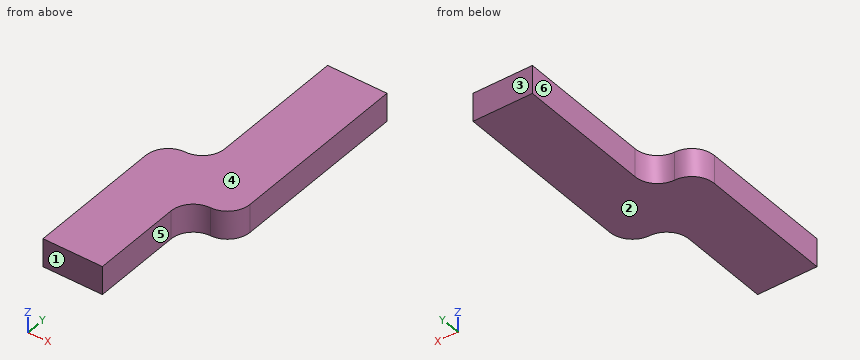
from build123d import *

# Parameters (mm, degrees)
F1_DEPTH = 6.3


with BuildPart() as f1:
    # F0 (on Top) → F1 (new body)
    with BuildSketch(Plane.XY):
        with BuildLine():
            Line((0, 30), (0, 0))
            Line((0, 0), (13.2, 0))
            Line((13.2, 0), (13.2, 20))
            ThreePointArc((13.2, 20), (14.664466, 23.535534), (18.2, 25))
            ThreePointArc((18.2, 25), (21.735534, 26.464466), (23.2, 30))
            Line((23.2, 30), (23.2, 70))
            Line((23.2, 70), (10, 70))
            Line((10, 70), (10, 40))
            ThreePointArc((10, 40), (8.535534, 36.464466), (5, 35))
            ThreePointArc((5, 35), (1.464466, 33.535534), (0, 30))
        make_face()
    extrude(amount=F1_DEPTH)


solid = f1.part
The listing builds one solid part. Answer for the finished solid, in the listing's coordinates (mm). Face numbers are marked on the shaded views. A direction names the side the tool comes from. Give positions to 0.01 mm unless a question says otherwise; leave off trailing zeros. Loops run counter-clockwise (first coordinate to the right, second up) from the corner with the lowest first, then second, coordinate; pieces in that order, holes last. Notation, with made-up numbers: (23, 5.25) - (61, 5.25) arc R11 ccw to (61, 10.25) - close; hole circle Ø5 at (0, 3.5). An arc over 180 degrees is marked (long way). Use one line per item in the form item = value.
1. Which of the six approach directions +Z, -Z, +X, -X, +Y, -Y give full straight-line access (tool end or side, diameter ignored) to the marked faces 4, 5 and 6?
Calculated:
face_4 = +Z, +X, -X, +Y, -Y
face_5 = +Z, -Z, +X, -Y
face_6 = +Z, -Z, -X, +Y
2. Section C-C on x = 3.25 is taken. Give the vertices of the cut face in (y, z).
Calculated:
outline = (0, 0) - (34.68, 0) - (34.68, 6.3) - (0, 6.3) - close
3. The mould has two halves that part along Y. Classify the marked faces 1, 2 and 3: pulls with the +Y half, pulls with the -Y half, needs draft (parallel to the pull), parting line crosses it, or undercut.
Calculated:
face_1 = pulls with the -Y half
face_2 = needs draft
face_3 = pulls with the +Y half
4. Given pin 1 Ø3 at (y, z) = (14.5, 4) entering from +X; pin 2 Ø2 at (y, z) = (51.5, 2) entering from -X, each flat-ended and moving along its own axis, determine where each tip first touches the part or whether it passes through.
Calculated:
pin_1 = 13.2
pin_2 = 10
5. Section A-A on z = 2.25 is taken. Give the vertices of the cut face in (x, y).
Calculated:
outline = (0, 0) - (13.2, 0) - (13.2, 20) arc R5 cw to (18.2, 25) arc R5 ccw to (23.2, 30) - (23.2, 70) - (10, 70) - (10, 40) arc R5 cw to (5, 35) arc R5 ccw to (0, 30) - close
6. Find the intervals of material crossed by line 1 along X through (y, z) = (60.5, 2.75); line 2 along X through (y, z) = (4, 2.5); line 3 along Y through (x, z) = (6.25, 6.25), in increasing order. Write a range as [from, to].
Calculated:
line_1 = [10, 23.2]
line_2 = [0, 13.2]
line_3 = [0, 35.16]
7. Section B-B on y = 11 is taken. Give the vertices of the cut face in (x, z).
Calculated:
outline = (0, 0) - (13.2, 0) - (13.2, 6.3) - (0, 6.3) - close
